The figure shows three views and two pictorial views of one solid part (mm, origin at its lowest corner). Answer the questions. A direction names the side the tool comes from. Coordinates: 2 decimals unless noted, no trailing zeros. Order: outer loops, then holes, each group sorted by start corner. A loop starts at its lowest first (then second) coordinate and runs counter-clockwise, first axis right, second up. Notation, with made-up numbers: (47.5, 25.5) -> (61.5, 25.5) arc R10 cw to (61.5, 30.5) -> close; hole circle Ø9 at (51.5, 44). An arc over 180 degrees is marked (long way). Write item = value, one per line. Start each with the question number.
Q1. Straight lines are drawn through the part: L1, parallel to Y at x = 32.85, z = 6.5; L2, parallel to X at y = 14.25, z = 2.5; L3, parallel to Z at x = 25, y = 4. For each, find the intervals that lie inside material, in ascending order. Write a range as from..to.
Q2. The part is cut by section B-B, the plane y = 7.5. Determine the outline of the cut face in (x, z), plus the area to 3 significant figures.
Q3. Flat-ended cylindrical pins translate along their axes: pin 1 (1.5 mm diameter, centred on x = 6, z = 14.5, fed in from +Y); pin 2 (1 mm diameter, centred on y = 7, z = 8.5, fed in from -X); pin 3 (8 mm diameter, centred on y = 10.5, z = 16.5, fed in from -X); pin 4 (1 mm diameter, centred on y = 6, z = 18, fed in from -X). Find the tip coordinate at first contact, or state that the pin passes through.
Q4. The part is cut by section C-C, the plane x = 27.5. Determine the outline of the cut face in (y, z), plus the area to 3 significant figures.
Q5. The part is cut by section A-A, the plane z = 6.5. Determine the outline of the cut face in (x, y), plus the area to 3 significant figures.
Q6. Which of the six approach directions +Z, -Z, +X, -X, +Y, -Y give full straight-line access (tool end or side, diameter ignored) to the marked faces 1 and 2?
Q7. The part is cut by section D-D, the plane y = 5. Determine the outline of the cut face in (x, z).
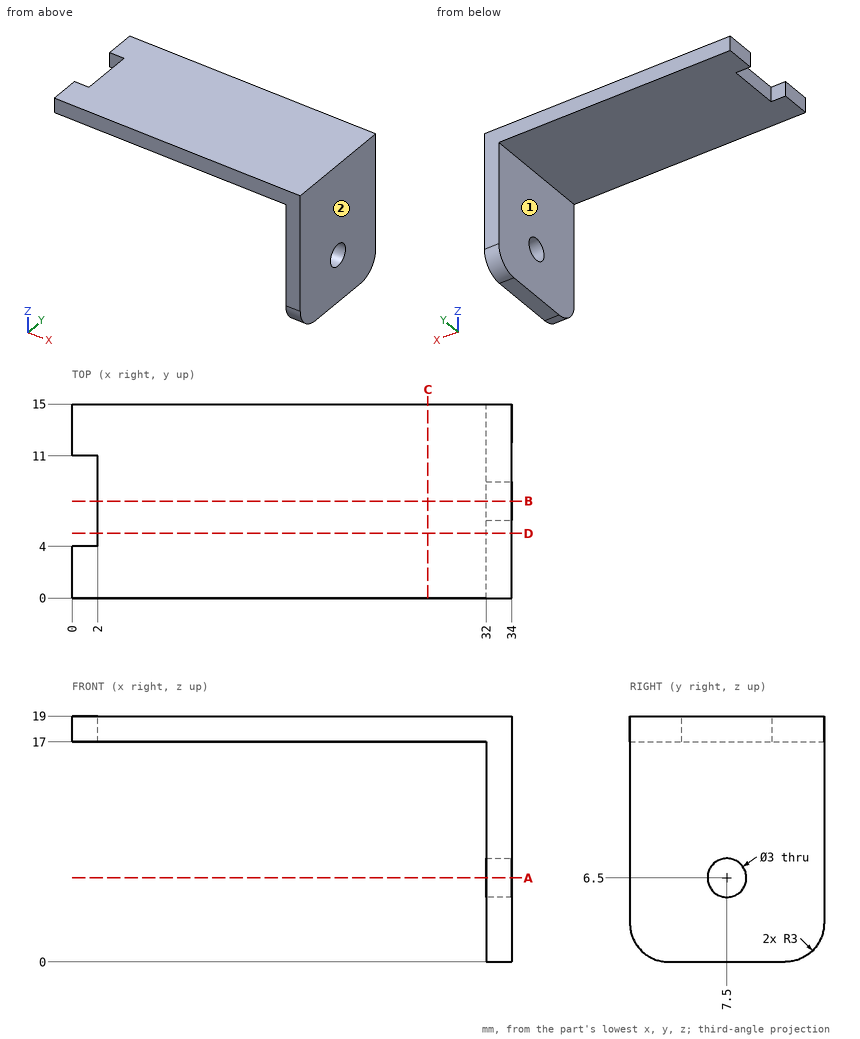
Model answer:
q1.L1 = 0..6, 9..15
q1.L2 = 32..34
q1.L3 = 17..19
q2.outline = (2, 17) -> (32, 17) -> (32, 8) -> (34, 8) -> (34, 19) -> (2, 19) -> close; (32, 0) -> (34, 0) -> (34, 5) -> (32, 5) -> close
q2.area = 92.0 mm2
q3.pin_1 = through
q3.pin_2 = 32
q3.pin_3 = 0
q3.pin_4 = 2
q4.outline = (0, 17) -> (15, 17) -> (15, 19) -> (0, 19) -> close
q4.area = 30.0 mm2
q5.outline = (32, 0) -> (34, 0) -> (34, 6) -> (32, 6) -> close; (32, 9) -> (34, 9) -> (34, 15) -> (32, 15) -> close
q5.area = 24.0 mm2
q6.face_1 = -Z, -X, +Y, -Y
q6.face_2 = +Z, -Z, +X, +Y, -Y
q7.outline = (2, 17) -> (32, 17) -> (32, 0) -> (34, 0) -> (34, 19) -> (2, 19) -> close
